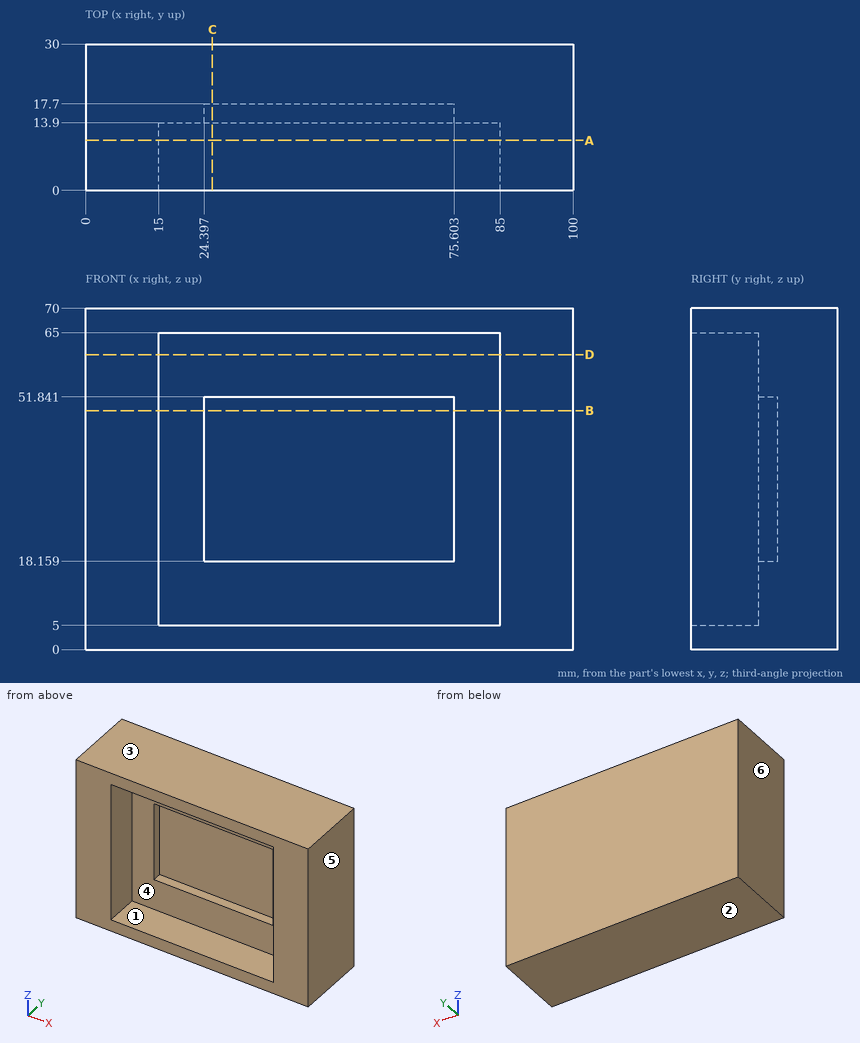
Print and shaded views of the part. All mm, measured from the part's lowest x, y and z. A direction names the side the tool comes from. Give positions to 0.01 mm unless a question says otherwise; leave off trailing zeros. Write each loop counter-clockwise with the first axis right and the second up, starting at its lowest first coordinate (ties: lowest second). Pieces come first, ordered by that corner, then holes. Notation, with made-up numbers: (-23.75, 40.25) - (1.25, 40.25) arc R17 cw to (1.25, 45.25) - close; hole circle Ø2 at (-16, 13.25). An arc over 180 degrees is marked (long way). Put each result on its own line as item: value.
(1) Tool access for the marked faces 1 and 2: list every direction of +Z, -Z, +X, -X, +Y, -Y with a clear straight run to the whole face (end or side of a thin tool).
Working result:
face 1: -Y
face 2: -Z, +X, -X, +Y, -Y
(2) Wall check: L1, parallel to Z at x = 43, y = 15; L2, parallel to X at y = 2, z = 53.5; L3, parallel to Z at x = 39, y = 5. Give the ranges that are in metal, low to high.
Working result:
L1: 0 to 18.16, 51.84 to 70
L2: 0 to 15, 85 to 100
L3: 0 to 5, 65 to 70
(3) Pull direction X, two halves, no side cores. Call the marked faces 3, 4, 5 and 6: released by +X, released by -X, zero draft, split by the parting line, or undercut.
Working result:
face 3: zero draft
face 4: undercut
face 5: released by +X
face 6: released by -X
(4) Saw through at C-C (x = 26). List the corners of the cut face in (y, z), then the cut area to 3 significant figures.
Working result:
outline: (0, 0) - (30, 0) - (30, 70) - (0, 70) - (0, 65) - (13.9, 65) - (13.9, 51.84) - (17.7, 51.84) - (17.7, 18.16) - (13.9, 18.16) - (13.9, 5) - (0, 5) - close
area: 1,140 mm^2
(5) Saw through at A-A (y = 10.25). List the corners of the cut face in (x, z), then the cut area to 3 significant figures.
Working result:
outline: (0, 0) - (100, 0) - (100, 70) - (0, 70) - close; hole (15, 5) - (85, 5) - (85, 65) - (15, 65) - close
area: 2,800 mm^2
(6) Drop a flat-ended pin along its axis: pin 1 Ø17 at (x, z) = (52, 43.5) entering from -Y. Give the stop position or say it passes through.
Working result:
pin 1: y = 13.9
(7) Saw through at B-B (z = 49). List the corners of the cut face in (x, y).
Working result:
outline: (0, 0) - (15, 0) - (15, 13.9) - (24.4, 13.9) - (24.4, 17.7) - (75.6, 17.7) - (75.6, 13.9) - (85, 13.9) - (85, 0) - (100, 0) - (100, 30) - (0, 30) - close
(8) Saw through at D-D (z = 60.5). List the corners of the cut face in (x, y).
Working result:
outline: (0, 0) - (15, 0) - (15, 13.9) - (85, 13.9) - (85, 0) - (100, 0) - (100, 30) - (0, 30) - close
